For this review, take the finished solid that the model builds, in its own axes (mm). Face numbers are marked on the shaded views. A direction names the side the tool comes from. Give positions to 0.01 mm unless a question says otherwise; leave off trailing zeros. Order: outer loops, then holes, each group sorted by start corner. A loop starts at its lowest first (then second) coordinate and runs counter-clockwise, first axis right, second up. Notation, with made-up numbers: (1.5, 40) -> (46.5, 40) arc R18 ccw to (46.5, 54) -> close; hole circle Ø3 at (7.25, -6.75). An arc over 180 degrees is marked (long way). Return JSON: item names as keys, results as strings. Group by question number.
1) For the marked faces 1 and 2, list the 3-axis set-ups (+Z, -Z, +X, -X, +Y, -Y) from which the entire face can be reached by the end or side of a thin tool; tool diameter is ignored.
2) Add section B-B (x = -56.5). Give the boundary of the cut face in (y, z).
3) Add section A-A (z = -3.5). Give the boundary of the cut face in (x, y).
4) Insertion check: P1, Ø5.5, axis at x = -58, y = 116.5, coming from the -Z side; P2, Ø9, axis at x = -48, y = 116.5, coming from the -Z side; P3, Ø0.6, axis at x = -55, z = -3.5, coming from the +Y side; P4, Ø1.7, axis at x = -53, z = -1.5, coming from the +Y side. Each pin has a flat end and moves straight along its axis. Give the tip position at first contact, or say it passes through.
5) To check wall thickness, follow line 1 along X through (y, z) = (113, -4.3); line 2 along X through (y, z) = (125, -2.45); line 3 along Z through (x, y) = (-57.25, 106.5). State the ranges of each line that lie inside material, in increasing order.
6) The part is to be moulded in two halves that separate along Y. For the marked faces 3 and 4, say which applies: released by +Y, released by -Y, zero draft, split by the parting line, or undercut.
from build123d import *

# Parameters (mm, degrees)
BOSS_EXTRUDE1_DEPTH = 2
BOSS_EXTRUDE2_DEPTH = 5
SKETCH6_W           = 20.1
SKETCH6_H           = 20.1
CUT_EXTRUDE1_DEPTH  = 3
SKETCH5_R           = 0.6
FILLET1_R           = 0.5


with BuildPart() as part:
    # Sketch2 → Boss-Extrude1 (new body)
    with BuildSketch(Plane.XY):
        with BuildLine():
            ThreePointArc((-60.960758129, 127.051811933), (-61.460758129, 127.185786529), (-61.826783532, 127.551811933))
            Line((-61.826783532, 127.551811933), (-67.460758129, 127.551811933))
            ThreePointArc((-67.460758129, 127.551811933), (-68.874971691, 126.966025495), (-69.460758129, 125.551811933))
            Line((-69.460758129, 125.551811933), (-69.460758129, 99.551811933))
            ThreePointArc((-69.460758129, 99.551811933), (-68.874971691, 98.13759837), (-67.460758129, 97.551811933))
            Line((-67.460758129, 97.551811933), (-41.460758129, 97.551811933))
            ThreePointArc((-41.460758129, 97.551811933), (-40.046544566, 98.13759837), (-39.460758129, 99.551811933))
            Line((-39.460758129, 99.551811933), (-39.460758129, 125.551811933))
            ThreePointArc((-39.460758129, 125.551811933), (-40.046544566, 126.966025495), (-41.460758129, 127.551811933))
            Line((-41.460758129, 127.551811933), (-47.094732725, 127.551811933))
            ThreePointArc((-47.094732725, 127.551811933), (-47.460758129, 127.185786529), (-47.960758129, 127.051811933))
            Line((-47.960758129, 127.051811933), (-60.960758129, 127.051811933))
        make_face()
    extrude(amount=-BOSS_EXTRUDE1_DEPTH)

    # Sketch2<2> → Boss-Extrude2 (add)
    with BuildSketch(Plane.XY):
        with BuildLine():
            Line((-65.460758129, 99.501811933), (-43.460758129, 99.501811933))
            ThreePointArc((-43.460758129, 99.501811933), (-42.011189227, 100.102243031), (-41.410758129, 101.551811933))
            Line((-41.410758129, 101.551811933), (-41.410758129, 123.551811933))
            ThreePointArc((-41.410758129, 123.551811933), (-42.011189227, 125.001380834), (-43.460758129, 125.601811933))
            Line((-43.460758129, 125.601811933), (-65.460758129, 125.601811933))
            ThreePointArc((-65.460758129, 125.601811933), (-66.91032703, 125.001380834), (-67.510758129, 123.551811933))
            Line((-67.510758129, 123.551811933), (-67.510758129, 101.551811933))
            ThreePointArc((-67.510758129, 101.551811933), (-66.91032703, 100.102243031), (-65.460758129, 99.501811933))
        make_face()
    extrude(amount=-BOSS_EXTRUDE2_DEPTH)

    # Sketch6 → Cut-Extrude1 (cut)
    with BuildSketch(Plane(origin=(0, 0, -5), x_dir=(-1, 0, 0), z_dir=(0, 0, -1))):
        with Locations((54.460758129, 112.551811933)):
            Rectangle(SKETCH6_W, SKETCH6_H)
    extrude(amount=-CUT_EXTRUDE1_DEPTH, mode=Mode.SUBTRACT)

    # Cut-Sweep1: sweep along a path in Sketch4
    with BuildLine(Plane.XY.offset(-3.5)) as cut_sweep1_path:
        Line((-41.410758129, 101.551811933), (-41.410758129, 123.551811933))
        ThreePointArc((-41.410758129, 123.551811933), (-42.011189227, 125.001380834), (-43.460758129, 125.601811933))
        Line((-43.460758129, 125.601811933), (-65.460758129, 125.601811933))
        ThreePointArc((-65.460758129, 125.601811933), (-66.91032703, 125.001380834), (-67.510758129, 123.551811933))
        Line((-67.510758129, 123.551811933), (-67.510758129, 101.551811933))
        ThreePointArc((-67.510758129, 101.551811933), (-66.91032703, 100.102243031), (-65.460758129, 99.501811933))
        Line((-65.460758129, 99.501811933), (-43.460758129, 99.501811933))
        ThreePointArc((-43.460758129, 99.501811933), (-42.011189227, 100.102243031), (-41.410758129, 101.551811933))
    # Sketch5 → Cut-Sweep1 (sweep, cut)
    with BuildSketch(Plane(origin=(-54.460758129, 0, 0), x_dir=(0, 0, -1), z_dir=(1, 0, 0))):
        with Locations((3.5, 125.601811933)):
            Circle(SKETCH5_R)
    sweep(path=cut_sweep1_path.line, mode=Mode.SUBTRACT)

    # Fillet1
    fillet1_edges = [part.edges().sort_by_distance(p)[0] for p in [
        (-44.277745427, 127.551811933, 0),
        (-40.046544566, 126.966025495, 0),
        (-39.460758129, 112.551811933, 0),
        (-40.046544566, 98.13759837, 0),
        (-54.460758129, 97.551811933, 0),
        (-68.874971691, 98.13759837, 0),
        (-69.460758129, 112.551811933, 0),
        (-68.874971691, 126.966025495, 0),
        (-64.64377083, 127.551811933, 0),
        (-61.460758129, 127.185786529, 0),
        (-54.460758129, 127.051811933, 0),
        (-47.460758129, 127.185786529, 0),
        (-64.510758129, 112.551811933, -2),
        (-54.460758129, 102.501811933, -2),
        (-44.410758129, 112.551811933, -2),
        (-54.460758129, 122.601811933, -2),
        (-42.011189227, 125.001380834, -5),
        (-54.460758129, 125.601811933, -5),
        (-66.91032703, 125.001380834, -5),
        (-67.510758129, 112.551811933, -5),
        (-66.91032703, 100.102243031, -5),
        (-54.460758129, 99.501811933, -5),
        (-42.011189227, 100.102243031, -5),
        (-41.410758129, 112.551811933, -5),
        (-64.510758129, 112.551811933, -5),
        (-54.460758129, 122.601811933, -5),
        (-44.410758129, 112.551811933, -5),
        (-54.460758129, 102.501811933, -5),
    ]]
    fillet(fillet1_edges, radius=FILLET1_R - 0.0001)  # a hair under: the kernel refuses the full size


solid = part.part
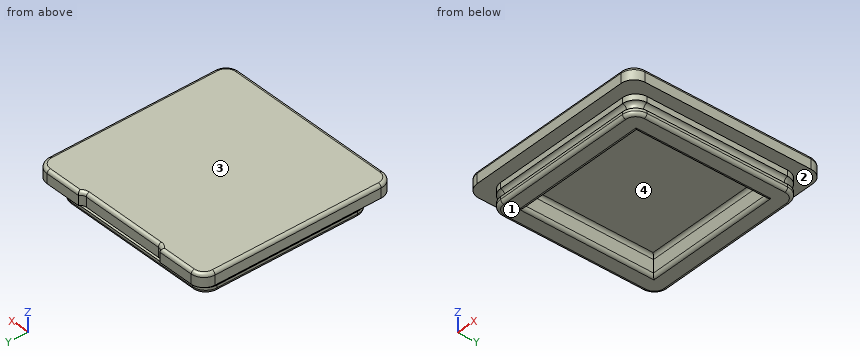
Evaluation:
{
 "1": {"face 1": "-Z, +X, -X, +Y, -Y", "face 2": "-Z"},
 "2": {"outline": "(97.55, -2) -> (99.5, -2) -> (99.5, -2.9) arc R0.6 cw to (99.5, -4.1) -> (99.5, -4.5) arc R0.5 ccw to (100, -5) -> (102, -5) arc R0.5 ccw to (102.5, -4.5) -> (102.5, -2.5) arc R0.5 cw to (103, -2) -> (122.1, -2) arc R0.5 cw to (122.6, -2.5) -> (122.6, -4.5) arc R0.5 ccw to (123.1, -5) -> (125.1, -5) arc R0.5 ccw to (125.6, -4.5) -> (125.6, -4.1) arc R0.6 cw to (125.6, -2.9) -> (125.6, -2) -> (127.05, -2) -> (127.05, -0.5) arc R0.5 ccw to (126.55, 0) -> (98.05, 0) arc R0.5 ccw to (97.55, -0.5) -> close"},
 "3": {"outline": "(-66.91, 101.55) arc R1.45 ccw to (-65.46, 100.1) -> (-43.46, 100.1) arc R1.45 ccw to (-42.01, 101.55) -> (-42.01, 123.55) arc R1.45 ccw to (-43.46, 125) -> (-65.46, 125) arc R1.45 ccw to (-66.91, 123.55) -> close; hole (-64.51, 102.5) -> (-44.41, 102.5) -> (-44.41, 122.6) -> (-64.51, 122.6) -> close"},
 "4": {"P1": "z = -2", "P2": "z = -5", "P3": "y = 125.08", "P4": "y = 127.05"},
 "5": {"line 1": "-67.51 to -64.51, -44.41 to -41.41", "line 2": "-66.91 to -42.01", "line 3": "-2 to 0"},
 "6": {"face 3": "zero draft", "face 4": "undercut"}
}
